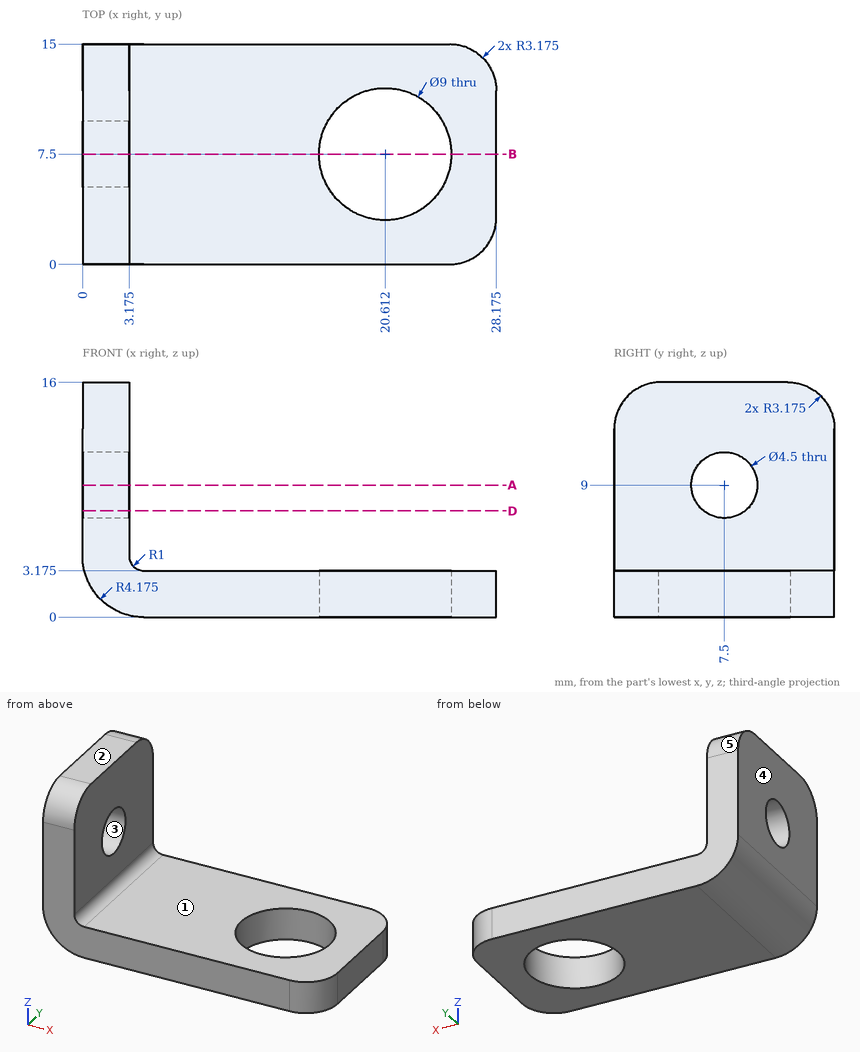
Design review of the part shown in the three views and the two pictorial views. Dimensions are in mm from the part's minimum x, y and z. A direction names the side the tool comes from. Give positions to 0.01 mm unless a question says otherwise; leave off trailing zeros. Loops run counter-clockwise (first coordinate to the right, second up) from the corner with the lowest first, then second, coordinate; pieces in that order, holes last. Notation, with made-up numbers: M -19,17 L -9,17 A14 cw -9,21 Z; hole C 69,-12 d2. An arc over 180 degrees is marked long. Answer as a JSON object with one key per item and string values. Group by question number.
Q1. Add section A-A on z = 9. Give the boundary of the cut face in (x, y) (3 decimals), and give its area (3 significant figures).
Q2. For probe 1 along Y at (x, z) = (0.8, 9); probe 2 along Z at (x, y) = (27, 9.5) (3 decimals), list the stretches that pass through material, from the lowest coordinate up. Write a range as [from, to].
Q3. Add section D-D on z = 7.25. Give the boundary of the cut face in (x, y) (3 decimals).
Q4. Insertion check: P1, Ø4, axis at y = 7, z = 8, coming from the +X side (3 decimals); P2, Ø6, axis at x = 8, y = 8.5, coming from the +Z side (3 decimals). Each pin has a flat end and moves straight along its axis. Give the tip position at first contact, or say it passes through.
Q5. Add section B-B on y = 7.5. Give the boundary of the cut face in (x, z) (3 decimals), and give its area (3 significant figures).
Q6. Tool access review of the marked faces 1 and 2: name each direction out of +Z, -Z, +X, -X, +Y, -Y from which nothing blocks a thin tool from reaching the whole face with its end or side.
Q7. Mouldability with a two-part tool opening along Z and no side actions: class the marked faces 3, 4 and 5 as +Z half, -Z half, draft (parallel to the pull), parting line (faces both ways), or undercut.
Checked values:
{
 "1": {"outline": "M 0,0 L 3.175,0 L 3.175,5.25 L 0,5.25 Z; M 0,9.75 L 3.175,9.75 L 3.175,15 L 0,15 Z", "area": "33.3 mm²"},
 "2": {"probe 1": "[0, 5.25], [9.75, 15]", "probe 2": "[0, 3.175]"},
 "3": {"outline": "M 0,0 L 3.175,0 L 3.175,6.086 L 0,6.086 Z; M 0,8.914 L 3.175,8.914 L 3.175,15 L 0,15 Z"},
 "4": {"P1": "x = 3.175", "P2": "z = 3.175"},
 "5": {"outline": "M 0,4.175 A4.175 ccw 4.175,0 L 16.112,0 L 16.112,3.175 L 4.175,3.175 A1 cw 3.175,4.175 L 3.175,6.75 L 0,6.75 Z; M 0,11.25 L 3.175,11.25 L 3.175,16 L 0,16 Z; M 25.112,0 L 28.175,0 L 28.175,3.175 L 25.112,3.175 Z", "area": "83.8 mm²"},
 "6": {"face 1": "+Z, +X, +Y, -Y", "face 2": "+Z, +X, -X, +Y, -Y"},
 "7": {"face 3": "undercut", "face 4": "draft", "face 5": "+Z half"}
}
